Here's how the part is built. I have some questions about the finished solid (model axes, mm). A direction names the side the tool comes from. Round coordinates to 2 decimals unless told otherwise and drop trailing zeros. Write each loop counter-clockwise with the first axis right and the second up, starting at its lowest first coordinate (ties: lowest second). Pieces come first, ordered by that corner, then holes. Notation, with made-up numbers: (40.5, 39) -> (94.5, 39) arc R34 ccw to (94.5, 75) -> close; hole circle Ø3 at (88.5, 68). An arc over 180 degrees is marked (long way). Put each result on its own line as item: value. Start each with the question number.
1) I want a section at D-D, the plane y = 6.5. List the corners of the cut face in (x, z) for me, then the cut area to 3 significant figures.
2) I want a section at B-B, the plane x = -2.75. List the corners of the cut face in (y, z) for me.
3) Will these pins go through, and if not, where does the flat tip stop? P1, Ø0.8, axis at x = 1, z = -2, coming from the -Y side; P2, Ø1.5, axis at x = -3.5, z = 0, coming from the -Y side.
4) We'd pull the mould along Z, two halves only. Please class faces 1 (the flat face through (6.15, 3, 0)), 2 (the flat face through (1.3, 6, 0.95)), 3 (the flat face through (0, 3, 2.9)): released by +Z, released by -Z, zero draft, split by the parting line, or undercut.
5) I want a section at A-A, the plane y = 2.5. List the corners of the cut face in (x, z) for me, then the cut area to 3 significant figures.
6) If I drill on line 1 along X through (y, z) = (0.75, -1.5); line 2 along Z through (x, y) = (4.75, 5.25); line 3 along Z through (x, y) = (-4, 6.25), over which ranges is the centre line in solid material (lowest first)? Write a range as [from, to].
7) I want a section at C-C, the plane z = 1.2. List the corners of the cut face in (x, y) for me, then the cut area to 3 significant figures.
8) Which directions (+Z, -Z, +X, -X, +Y, -Y) give clear straight access to the entire face, cutting with the end or side of a thin tool? Please do faces 4 (the flat face through (0, 3, -2.9)), 5 (the flat face through (0, 5, 1)), 6 (the flat face through (-4, 6, 0.95)).
from build123d import *

# Parameters (mm, degrees)
SKETCH1_W           = 12.3
SKETCH1_H           = 5.8
BOSS_EXTRUDE1_DEPTH = 7
SKETCH3_W           = 11
SKETCH3_H           = 4.9
CUT_EXTRUDE1_DEPTH  = 5
SKETCH4_W           = 1.2
SKETCH4_H           = 3.5
CUT_EXTRUDE2_DEPTH  = 4
SKETCH5_W           = 12.3
SKETCH5_H           = 0.8
CUT_EXTRUDE3_DEPTH  = 0.8
SKETCH6_W           = 0.8
SKETCH6_H           = 0.8
CUT_EXTRUDE4_DEPTH  = 10
SKETCH7_W           = 11
SKETCH7_H           = 1
CUT_EXTRUDE5_DEPTH  = 0.3


with BuildPart() as part:
    # Sketch1 → Boss-Extrude1 (new body)
    with BuildSketch(Plane(origin=(0, 0, 0), x_dir=(1, 0, 0), z_dir=(0, 1, 0))):
        Rectangle(SKETCH1_W, SKETCH1_H)
    extrude(amount=BOSS_EXTRUDE1_DEPTH)

    # Sketch3 → Cut-Extrude1 (cut)
    with BuildSketch(Plane.XZ):
        Rectangle(SKETCH3_W, SKETCH3_H)
    extrude(amount=-CUT_EXTRUDE1_DEPTH, mode=Mode.SUBTRACT)

    # Sketch4 → Cut-Extrude2 (cut)
    with BuildSketch(Plane.XY.offset(2.9)):
        with Locations((-3.56, 1.75)):
            Rectangle(SKETCH4_W, SKETCH4_H)
        with Locations((3.24, 1.75)):
            Rectangle(SKETCH4_W, SKETCH4_H)
    extrude(amount=-CUT_EXTRUDE2_DEPTH, mode=Mode.SUBTRACT)

    # Sketch5 → Cut-Extrude3 (cut)
    with BuildSketch(Plane(origin=(0, 7, 0), x_dir=(1, 0, 0), z_dir=(0, 1, 0))):
        with Locations((0, 2.5)):
            Rectangle(SKETCH5_W, SKETCH5_H)
    extrude(amount=-CUT_EXTRUDE3_DEPTH, mode=Mode.SUBTRACT)

    # Sketch6 → Cut-Extrude4 (cut)
    with BuildSketch(Plane(origin=(0, 7, 0), x_dir=(1, 0, 0), z_dir=(0, 1, 0))):
        with Locations((3.8, -0.55)):
            Rectangle(SKETCH6_W, SKETCH6_H)
        with Locations((-1.266666667, -0.55)):
            Rectangle(SKETCH6_W, SKETCH6_H)
        with Locations((1.266666667, -0.55)):
            Rectangle(SKETCH6_W, SKETCH6_H)
        with Locations((-3.8, -0.55)):
            Rectangle(SKETCH6_W, SKETCH6_H)
    extrude(amount=-CUT_EXTRUDE4_DEPTH, mode=Mode.SUBTRACT)

    # Sketch7 → Cut-Extrude5 (cut)
    with BuildSketch(Plane.XZ.offset(-5)):
        with Locations((0, -1.95)):
            Rectangle(SKETCH7_W, SKETCH7_H)
    extrude(amount=-CUT_EXTRUDE5_DEPTH, mode=Mode.SUBTRACT)


solid = part.part
Findings:
1. outline: (-6.15, -2.1) -> (6.15, -2.1) -> (6.15, 2.9) -> (-6.15, 2.9) -> close; hole (-4.2, 0.15) -> (-3.4, 0.15) -> (-3.4, 0.95) -> (-4.2, 0.95) -> close; hole (-1.67, 0.15) -> (-0.87, 0.15) -> (-0.87, 0.95) -> (-1.67, 0.95) -> close; hole (0.87, 0.15) -> (1.67, 0.15) -> (1.67, 0.95) -> (0.87, 0.95) -> close; hole (3.4, 0.15) -> (4.2, 0.15) -> (4.2, 0.95) -> (3.4, 0.95) -> close
1. area: 58.9 mm2
2. outline: (0, -2.9) -> (6.2, -2.9) -> (6.2, -2.1) -> (7, -2.1) -> (7, 2.9) -> (0, 2.9) -> (0, 2.45) -> (5, 2.45) -> (5, -1.45) -> (5.3, -1.45) -> (5.3, -2.45) -> (0, -2.45) -> close
3. P1: stops at y = 5.3
3. P2: stops at y = 5
4. face 1: zero draft
4. face 2: undercut
4. face 3: released by +Z
5. outline: (-6.15, -2.9) -> (6.15, -2.9) -> (6.15, 2.9) -> (3.84, 2.9) -> (3.84, 2.45) -> (5.5, 2.45) -> (5.5, -2.45) -> (-5.5, -2.45) -> (-5.5, 2.45) -> (-4.16, 2.45) -> (-4.16, 2.9) -> (-6.15, 2.9) -> close; (-2.96, 2.45) -> (2.64, 2.45) -> (2.64, 2.9) -> (-2.96, 2.9) -> close
5. area: 16.4 mm2
6. line 1: x = [-6.15, -5.5], [5.5, 6.15]
6. line 2: z = [-2.9, -2.45], [-1.45, 2.9]
6. line 3: z = [-2.1, 0.15], [0.95, 2.9]
7. outline: (-6.15, 0) -> (-5.5, 0) -> (-5.5, 5) -> (5.5, 5) -> (5.5, 0) -> (6.15, 0) -> (6.15, 7) -> (-6.15, 7) -> close
7. area: 31.1 mm2
8. face 4: -Z, +X, -X, +Y, -Y
8. face 5: -Y
8. face 6: +Y, -Y
